The listing builds one solid part. Answer for the finished solid, in the listing's coordinates (mm). Face numbers are marked on the shaded views. A direction names the side the tool comes from. Give positions to 0.01 mm unless a question says otherwise; leave off trailing zeros. Write each loop counter-clockwise with the first axis right and the second up, starting at its lowest first coordinate (ties: lowest second). Pieces come first, ordered by that corner, then holes. Notation, with made-up numbers: (83.25, 20) -> (135.25, 20) arc R22 ccw to (135.25, 54) -> close; hole circle Ø1 at (60, 83). An arc over 180 degrees is marked (long way). One line per question, with ' | ' between items.
from build123d import *

# Parameters (mm, degrees)
F0_R     = 1.6
F0_W     = 6
F0_H     = 4
F1_DEPTH = 1.6
F2_W     = 5.5
F2_H     = 4.5
F3_DEPTH = 1.2
F2_W_2   = 7.5
F2_H_2   = 15.5
F4_DEPTH = 2.65
F2_R     = 0.635
F2_R_2   = 0.3175
F5_DEPTH = 25
F6_W     = 8.5
F6_H     = 8.5
F7_DEPTH = 11.9
F6_W_2   = 2
F6_H_2   = 2.25
F8_DEPTH = 0.8
F6_W_3   = 3
F6_H_3   = 3.25
F9_DEPTH = 1.1


with BuildPart() as f1:
    # F0 (on Top) → F1 (new body)
    with BuildSketch(Plane.XY):
        Polygon((-15, 15), (-15, -15), (27.5, -15), (33.5, -9), (33.5, 9), (27.5, 15), align=None)
        with Locations((-12, -12)):
            Circle(F0_R, mode=Mode.SUBTRACT)
        with Locations((12, -12)):
            Circle(F0_R, mode=Mode.SUBTRACT)
        with BuildLine():
            ThreePointArc((10, 9.7979589711), (12.5492658483, 6.2061200978), (13.8564064606, 2))
            Line((13.8564064606, 2), (14, 2))
            Line((14, 2), (14, 0))
            Line((14, 0), (14, -2))
            Line((14, -2), (13.8564064606, -2))
            ThreePointArc((13.8564064606, -2), (12.5492658483, -6.2061200978), (10, -9.7979589711))
            ThreePointArc((10, -9.7979589711), (-14, 0), (10, 9.7979589711))
        make_face(mode=Mode.SUBTRACT)
        with Locations((-12, 12)):
            Circle(F0_R, mode=Mode.SUBTRACT)
        with Locations((12, 12)):
            Circle(F0_R, mode=Mode.SUBTRACT)
        Polygon((4, 2), (4, 4), (-4, 4), (-4, -4), (4, -4), (4, -2), align=None)
        with Locations((7, 0)):
            Rectangle(F0_W, F0_H)
        with BuildLine():
            Line((10, 9.7979589711), (10, 2))
            Line((10, 2), (13.8564064606, 2))
            ThreePointArc((13.8564064606, 2), (12.5492658483, 6.2061200978), (10, 9.7979589711))
        make_face()
        with BuildLine():
            Line((13.8564064606, -2), (10, -2))
            Line((10, -2), (10, -9.7979589711))
            ThreePointArc((10, -9.7979589711), (12.5492658483, -6.2061200978), (13.8564064606, -2))
        make_face()
        with BuildLine():
            Line((13.8564064606, 2), (10, 2))
            Line((10, 2), (10, -2))
            Line((10, -2), (13.8564064606, -2))
            ThreePointArc((13.8564064606, -2), (13.964055472, -1.0025740751), (14, 0))
            ThreePointArc((14, 0), (13.964055472, 1.0025740751), (13.8564064606, 2))
        make_face()
        with BuildLine():
            Line((14, 2), (13.8564064606, 2))
            ThreePointArc((13.8564064606, 2), (13.964055472, 1.0025740751), (14, 0))
            Line((14, 0), (14, 2))
        make_face()
        with BuildLine():
            ThreePointArc((14, 0), (13.964055472, -1.0025740751), (13.8564064606, -2))
            Line((13.8564064606, -2), (14, -2))
            Line((14, -2), (14, 0))
        make_face()
    extrude(amount=F1_DEPTH)

    # F2 (on face) → F3 (join)
    with BuildSketch(Plane.XY.offset(1.6)):
        Rectangle(F2_W, F2_H)
    extrude(amount=F3_DEPTH)

    # F2 (on face) → F4 (join)
    with BuildSketch(Plane.XY.offset(1.6)):
        with Locations((21.5, 5)):
            Rectangle(F2_W_2, F2_H_2)
    extrude(amount=F4_DEPTH)

    # F2 (on face) → F5 (cut)
    with BuildSketch(Plane.XY.offset(1.6)):
        with Locations((18.96, -4.125)):
            Circle(F2_R)
        with Locations((21.5, -4.125)):
            Circle(F2_R)
        with Locations((24.04, -4.125)):
            Circle(F2_R)
        with Locations((19.645, -6.1875)):
            Circle(F2_R_2)
        with Locations((18.375, -6.1875)):
            Circle(F2_R_2)
        with Locations((29.3125, -7.625)):
            Circle(F2_R)
        with Locations((31.8525, -7.625)):
            Circle(F2_R)
        with Locations((31.8525, -5.085)):
            Circle(F2_R)
        with Locations((29.3125, -5.085)):
            Circle(F2_R)
        with Locations((29.3125, -2.545)):
            Circle(F2_R)
        with Locations((31.8525, -2.545)):
            Circle(F2_R)
        with Locations((31.8525, -0.005)):
            Circle(F2_R)
        with Locations((29.3125, -0.005)):
            Circle(F2_R)
        with Locations((29.3125, 2.535)):
            Circle(F2_R)
        with Locations((31.8525, 2.535)):
            Circle(F2_R)
        with Locations((31.8525, 5.075)):
            Circle(F2_R)
        with Locations((29.3125, 5.075)):
            Circle(F2_R)
        with Locations((29.3125, 7.615)):
            Circle(F2_R)
        with Locations((31.8525, 7.615)):
            Circle(F2_R)
    extrude(amount=-F5_DEPTH, mode=Mode.SUBTRACT)

    # F6 (on face) → F7 (join)
    with BuildSketch(Plane(origin=(0, 0, 0), x_dir=(1, 0, 0), z_dir=(0, 0, -1))):
        with Locations((22.75, -10.5)):
            Rectangle(F6_W, F6_H)
    extrude(amount=F7_DEPTH)

    # F6 (on face) → F8 (join)
    with BuildSketch(Plane(origin=(0, 0, 0), x_dir=(1, 0, 0), z_dir=(0, 0, -1))):
        with Locations((19, 9.375)):
            Rectangle(F6_W_2, F6_H_2)
    extrude(amount=F8_DEPTH)

    # F6 (on face) → F9 (join)
    with BuildSketch(Plane(origin=(0, 0, 0), x_dir=(1, 0, 0), z_dir=(0, 0, -1))):
        with Locations((25.25, 9.375)):
            Rectangle(F6_W_3, F6_H_3)
    extrude(amount=F9_DEPTH)


solid = f1.part
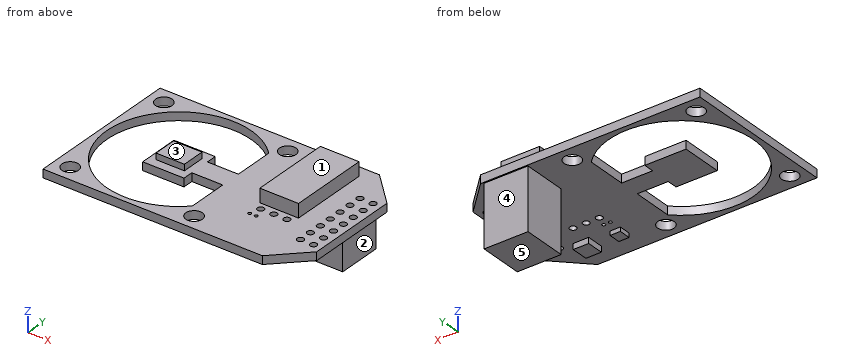
Item 1: Consider line 1 (Y direction, x = -12, z = 0.4); line 2 (Y direction, x = 5, z = 1); line 3 (Z direction, x = -2, y = 0). Determine where each line is inside the solid, lowest interval first. Write a range as [from, to].
Answers below:
line 1: [-15, -13.6], [-10.4, -7.21], [7.21, 10.4], [13.6, 15] | line 2: [-15, -13.08], [-2, 2], [13.08, 15] | line 3: [0, 2.8]
Item 2: Find section A-A (x = 21.5). Write down the section's boundary in (y, z), then the cut area to 3 significant figures.
Answers below:
outline: (-15, 0) -> (-4.76, 0) -> (-4.76, 1.6) -> (-15, 1.6) -> close; (-3.49, 0) -> (6.25, 0) -> (6.25, -11.9) -> (14.75, -11.9) -> (14.75, 0) -> (15, 0) -> (15, 1.6) -> (12.75, 1.6) -> (12.75, 4.25) -> (-2.75, 4.25) -> (-2.75, 1.6) -> (-3.49, 1.6) -> close | area: 188 mm²
Item 3: Find section C-C (y = 12). Write down the section's boundary in (x, z).
Answers below:
outline: (-15, 0) -> (-13.6, 0) -> (-13.6, 1.6) -> (-15, 1.6) -> close; (-10.4, 0) -> (-7.21, 0) -> (-7.21, 1.6) -> (-10.4, 1.6) -> close; (7.21, 0) -> (10.4, 0) -> (10.4, 1.6) -> (7.21, 1.6) -> close; (13.6, 0) -> (18.5, 0) -> (18.5, -11.9) -> (27, -11.9) -> (27, 0) -> (30.5, 0) -> (30.5, 1.6) -> (25.25, 1.6) -> (25.25, 4.25) -> (17.75, 4.25) -> (17.75, 1.6) -> (13.6, 1.6) -> close
Item 4: Find section D-D (x = 0). Write down the section's boundary in (y, z).
Answers below:
outline: (-15, 0) -> (-14, 0) -> (-14, 1.6) -> (-15, 1.6) -> close; (-4, 0) -> (4, 0) -> (4, 1.6) -> (2.25, 1.6) -> (2.25, 2.8) -> (-2.25, 2.8) -> (-2.25, 1.6) -> (-4, 1.6) -> close; (14, 0) -> (15, 0) -> (15, 1.6) -> (14, 1.6) -> close
Item 5: Flat-ended cylindrical pins translate along their axes: pin 1 (1.5 mm diameter, centred on x = 31.85, y = -2.54, fed in from -Z); pin 2 (1.7 mm diameter, centred on x = 29.31, y = 0, fed in from +Z); pin 3 (15 mm diameter, centred on x = 9, y = -5.5, fed in from +Z). Find the tip coordinate at first contact, or state that the pin passes through.
Answers below:
pin 1: z = 0 | pin 2: z = 1.6 | pin 3: z = 2.8
Item 6: A tool of negligible diameter and unlimited length cuts with its end or side. For the marked faces 1, 2, 3, 4 and 5, from which of +Z, -Z, +X, -X, +Y, -Y can it reach the whole face along a straight path? Write none if from no direction.
Answers below:
face 1: +Z, +X, -X, +Y, -Y | face 2: -Z, +X, +Y, -Y | face 3: +Z, -X, +Y, -Y | face 4: -Z, +X, -X, +Y | face 5: -Z, +X, -X, +Y, -Y
Item 7: Find section B-B (x = 12). Write down the section's boundary in (y, z), then the cut area to 3 significant figures.
Answers below:
outline: (-15, 0) -> (-13.6, 0) -> (-13.6, 1.6) -> (-15, 1.6) -> close; (-10.4, 0) -> (10.4, 0) -> (10.4, 1.6) -> (-10.4, 1.6) -> close; (13.6, 0) -> (15, 0) -> (15, 1.6) -> (13.6, 1.6) -> close | area: 37.8 mm²
